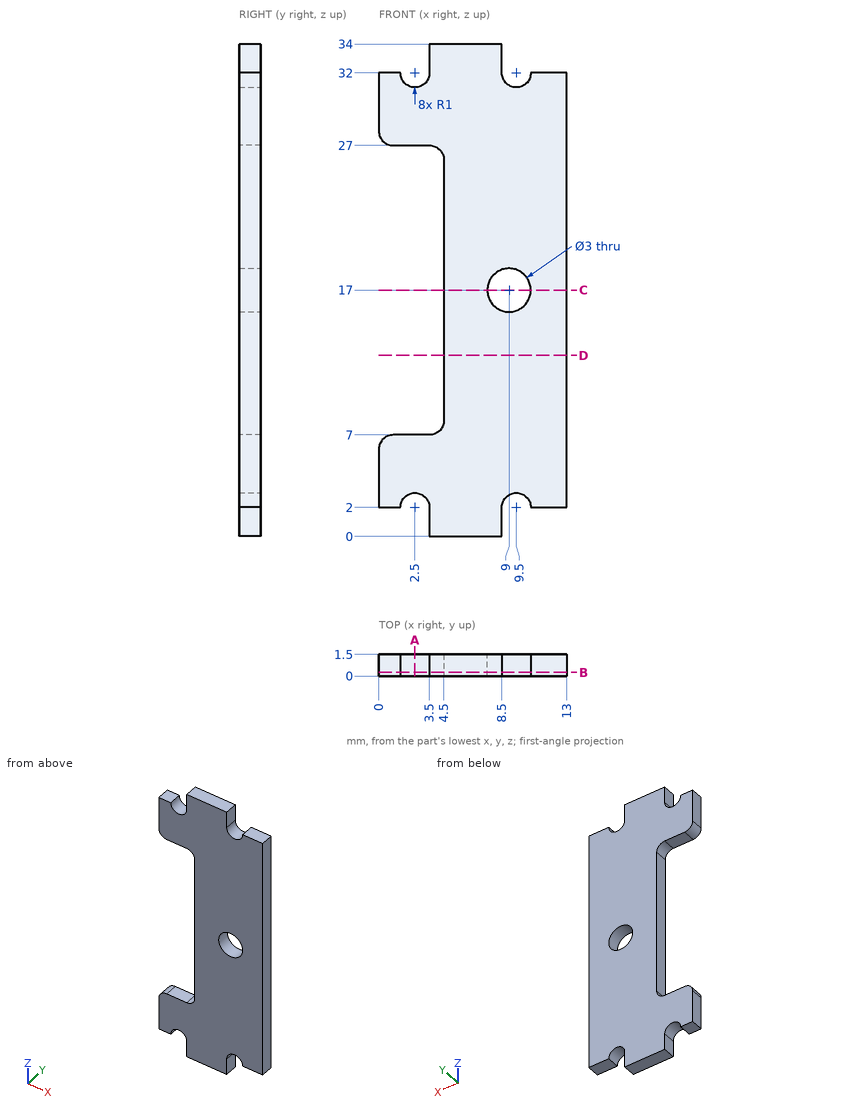
Could you check a few things on this drawing? It's one solid part, dimensions in mm from its lowest x, y, z. Give positions to 0.01 mm unless a question says otherwise; leave off trailing zeros. Order: outer loops, then holes, each group sorted by start corner. A loop starts at its lowest first (then second) coordinate and runs counter-clockwise, first axis right, second up. Notation, with made-up numbers: (34.5, -37.5) - (87.5, -37.5) arc R32 cw to (87.5, -2.5) - close; hole circle Ø9 at (19.25, -22). An arc over 180 degrees is marked (long way). Answer as a JSON object with one key per item and string values. Group by question number.
Item 1: If we section it at B-B on y = 0.25: Please give me the cut outline in (x, z), and give its area (3 significant figures).
Item 2: If we section it at C-C on z = 17: Please give me the cut outline in (x, y), and give its area (3 significant figures).
Item 3: Please list where these lines run through material, in increasing order: probe 1 along Z at (x, y) = (11.5, 0.1); probe 2 along X at (y, z) = (0.7, 11); probe 3 along Z at (x, y) = (1.25, 0.8).
Item 4: For P1, Ø0.8, axis at y = 1, z = 19, coming from the -X side; P2, Ø0.8, axis at x = 1.5, y = 1, coming from the -Z side; P3, Ø0.8, axis at y = 1, z = 33, coming from the +X side; P4, Ø3.5, axis at x = 9, z = 17, coming from the -Y side, each with a flat end and sliding along its axis, tell me the tip position at first contact or that it passes through.
Item 5: If we section it at D-D on z = 12.5: Please give me the cut outline in (x, y), and give its area (4 significant figures).
Item 6: If we section it at A-A on x = 2.5: Please give me the cut outline in (y, z).
Result set:
{
 "1": {"outline": "(0, 2) - (1.5, 2) arc R1 cw to (3.5, 2) - (3.5, 0) - (8.5, 0) - (8.5, 2) arc R1 cw to (10.5, 2) - (13, 2) - (13, 32) - (10.5, 32) arc R1 cw to (8.5, 32) - (8.5, 34) - (3.5, 34) - (3.5, 32) arc R1 cw to (1.5, 32) - (0, 32) - (0, 28) arc R1 ccw to (1, 27) - (3.5, 27) arc R1 cw to (4.5, 26) - (4.5, 8) arc R1 cw to (3.5, 7) - (1, 7) arc R1 ccw to (0, 6) - close; hole circle Ø3 at (9, 17)", "area": "307 mm²"},
 "2": {"outline": "(4.5, 0) - (7.5, 0) - (7.5, 1.5) - (4.5, 1.5) - close; (10.5, 0) - (13, 0) - (13, 1.5) - (10.5, 1.5) - close", "area": "8.25 mm²"},
 "3": {"probe 1": "2 to 32", "probe 2": "4.5 to 13", "probe 3": "2 to 7, 27 to 32"},
 "4": {"P1": "x = 4.5", "P2": "z = 2", "P3": "x = 8.5", "P4": "y = 0"},
 "5": {"outline": "(4.5, 0) - (13, 0) - (13, 1.5) - (4.5, 1.5) - close", "area": "12.75 mm²"},
 "6": {"outline": "(0, 3) - (1.5, 3) - (1.5, 7) - (0, 7) - close; (0, 27) - (1.5, 27) - (1.5, 31) - (0, 31) - close"}
}
